Input: part model. Units: mm. Frame: model coordinates. A direction names the side the tool comes from. Round coordinates to 2 decimals unless told otherwise and drop trailing zeros. Write each loop counter-clockwise with the first axis right and the second up, starting at its lowest first coordinate (ties: lowest second). Pieces come first, ordered by that corner, then holes. Notation, with made-up numbers: (0, 6.25) - (47, 6.25) arc R21 cw to (47, 38.25) - close; hole circle Ø11 at (46.5, 14). An arc over 180 degrees is marked (long way). One line per item, written item: value. Start each with the question number.
```python
from build123d import *

# Parameters (mm, degrees)
BOX028_W          = 41.4
BOX028_H          = 10
BOX028_DEPTH      = 11
BOX028_ROLL_ANGLE = 45
BOX037_W          = 0.4
BOX037_H          = 27
BOX037_DEPTH      = 9
BOX036_W          = 0.4
BOX036_H          = 27
BOX036_DEPTH      = 9
BOX035_W          = 0.4
BOX035_H          = 27
BOX035_DEPTH      = 9
BOX034_W          = 0.4
BOX034_H          = 27
BOX034_DEPTH      = 9
BOX038_W          = 0.4
BOX038_H          = 27
BOX038_DEPTH      = 9
BOX033_W          = 36.4
BOX033_H          = 27
BOX033_DEPTH      = 0.4


with BuildPart() as rear_panel_chamfer:
    # Box028 → Box028 (new body)
    with BuildSketch(Plane.XY):
        with Locations((20.7, 5)):
            Rectangle(BOX028_W, BOX028_H)
    extrude(amount=BOX028_DEPTH)


with BuildPart() as rear_panel_chamfer_1:
    # Box028 roll: moved
    add(rear_panel_chamfer.part.rotate(Axis((0, 0, 0), (1, 0, 0)), BOX028_ROLL_ANGLE))


with BuildPart() as rear_panel_chamfer_2:
    # Box028 placement: moved
    add(rear_panel_chamfer_1.part.moved(Location((-21.6, 27, 12.81))))


with BuildPart() as support_y4_for_rear_panel_angled:
    # Box037 → Box037 (new body)
    with BuildSketch(Plane(origin=(-2.2, 0.1, 11.4), x_dir=(1, 0, 0), z_dir=(0, 0, 1))):
        with Locations((0.2, 13.5)):
            Rectangle(BOX037_W, BOX037_H)
    extrude(amount=BOX037_DEPTH)


with BuildPart() as support_y3_for_rear_panel_angled:
    # Box036 → Box036 (new body)
    with BuildSketch(Plane(origin=(4.8, 0.1, 11.4), x_dir=(1, 0, 0), z_dir=(0, 0, 1))):
        with Locations((0.2, 13.5)):
            Rectangle(BOX036_W, BOX036_H)
    extrude(amount=BOX036_DEPTH)


with BuildPart() as support_y2_for_rear_panel_angled:
    # Box035 → Box035 (new body)
    with BuildSketch(Plane(origin=(-8.2, 0.1, 11.4), x_dir=(1, 0, 0), z_dir=(0, 0, 1))):
        with Locations((0.2, 13.5)):
            Rectangle(BOX035_W, BOX035_H)
    extrude(amount=BOX035_DEPTH)


with BuildPart() as support_y1_for_rear_panel_angled:
    # Box034 → Box034 (new body)
    with BuildSketch(Plane(origin=(-14.2, 0.1, 11.4), x_dir=(1, 0, 0), z_dir=(0, 0, 1))):
        with Locations((0.2, 13.5)):
            Rectangle(BOX034_W, BOX034_H)
    extrude(amount=BOX034_DEPTH)


with BuildPart() as support_y5_for_rear_panel_angled:
    # Box038 → Box038 (new body)
    with BuildSketch(Plane(origin=(10.8, 0.1, 11.4), x_dir=(1, 0, 0), z_dir=(0, 0, 1))):
        with Locations((0.2, 13.5)):
            Rectangle(BOX038_W, BOX038_H)
    extrude(amount=BOX038_DEPTH)


with BuildPart() as supports_for_rear_panel_angled_chamfered:
    # Box033 → Box033 (new body)
    with BuildSketch(Plane(origin=(-19, 0.1, 11.4), x_dir=(1, 0, 0), z_dir=(0, 0, 1))):
        with Locations((18.2, 13.5)):
            Rectangle(BOX033_W, BOX033_H)
    extrude(amount=BOX033_DEPTH)

    # Fusion005: union support Y4 for rear panel angled, support Y3 for rear panel angled, support Y2 for rear panel angled, support Y1 for rear panel angled, support Y5 for rear panel angled
    add(support_y4_for_rear_panel_angled.part)
    add(support_y3_for_rear_panel_angled.part)
    add(support_y2_for_rear_panel_angled.part)
    add(support_y1_for_rear_panel_angled.part)
    add(support_y5_for_rear_panel_angled.part)

    # Cut006: cut Rear panel chamfer
    add(rear_panel_chamfer_2.part, mode=Mode.SUBTRACT)


solid = supports_for_rear_panel_angled_chamfered.part
```
Q1. Access query for faces 4 (the flat face through (8, 14, 11.8)), 5 (the flat face through (14, 14, 11.8)), 6 (the flat face through (-0.88, 0.1, 11.55)). Directions: +Z, -Z, +X, -X, +Y, -Y. A direction counts if a zero-diameter tool reaches every point of the face in a straight line with its end or side. Return the directions, or none.
Q2. Pull-direction query (X, two-part tool) for faces 1 (the flat face through (-17, 14, 11.8)), 2 (the flat face through (-11, 14, 11.8)), 3 (the flat face through (11.2, 13, 16)); classes: pulls with the +X half, pulls with the -X half, needs draft (parallel to the pull), parting line crosses it, or undercut.
Q3. Contact query for flat-ended pins moving along their axis: pin 1 Ø4.5 at (y, z) = (13.5, 14.5) entering from +X; pin 2 Ø1.7 at (x, y) = (-10.5, 19.5) entering from +Z; pin 3 Ø5 at (y, z) = (20, 13) entering from -X; pin 4 Ø1.5 at (x, z) = (12, 19) entering from +Y. Output: stop coordinate, or through.
Q4. Cut plane A-A, the plane z = 15.5. Output: boundary loops of the cut face in (x, y), and give its area (3 significant figures).
Q5. Cut plane D-D, the plane y = 17.75. Output: boundary loops of the cut face in (x, z).
Q6. Material intervals for probe 1 along X at (y, z) = (7.5, 15.5); probe 2 along Z at (x, y) = (-6.5, 12.5); probe 3 along Y at (x, z) = (-14, 15), sorted ascending. Write a range as from..to.
Q7. Cut plane B-B, the plane y = 23.25. Output: boundary loops of the cut face in (x, z), and give its area (3 significant figures).
Q8. Cut plane C-C, the plane z = 17.75. Output: boundary loops of the cut face in (x, y), and give its area (3 significant figures).
A:
1. face 4: +Z, +Y, -Y
1. face 5: +Z, +X, +Y, -Y
1. face 6: +Z, -Z, +X, -X, -Y
2. face 1: needs draft
2. face 2: undercut
2. face 3: pulls with the +X half
3. pin 1: stops at x = 11.2
3. pin 2: stops at z = 11.8
3. pin 3: stops at x = -19
3. pin 4: passes through
4. outline: (-14.2, 0.1) - (-13.8, 0.1) - (-13.8, 24.31) - (-14.2, 24.31) - close; (-8.2, 0.1) - (-7.8, 0.1) - (-7.8, 24.31) - (-8.2, 24.31) - close; (-2.2, 0.1) - (-1.8, 0.1) - (-1.8, 24.31) - (-2.2, 24.31) - close; (4.8, 0.1) - (5.2, 0.1) - (5.2, 24.31) - (4.8, 24.31) - close; (10.8, 0.1) - (11.2, 0.1) - (11.2, 24.31) - (10.8, 24.31) - close
4. area: 48.4 mm²
5. outline: (-19, 11.4) - (17.4, 11.4) - (17.4, 11.8) - (11.2, 11.8) - (11.2, 20.4) - (10.8, 20.4) - (10.8, 11.8) - (5.2, 11.8) - (5.2, 20.4) - (4.8, 20.4) - (4.8, 11.8) - (-1.8, 11.8) - (-1.8, 20.4) - (-2.2, 20.4) - (-2.2, 11.8) - (-7.8, 11.8) - (-7.8, 20.4) - (-8.2, 20.4) - (-8.2, 11.8) - (-13.8, 11.8) - (-13.8, 20.4) - (-14.2, 20.4) - (-14.2, 11.8) - (-19, 11.8) - close
6. probe 1: x = -14.2..-13.8, -8.2..-7.8, -2.2..-1.8, 4.8..5.2, 10.8..11.2
6. probe 2: z = 11.4..11.8
6. probe 3: y = 0.1..24.81
7. outline: (-19, 11.4) - (17.4, 11.4) - (17.4, 11.8) - (11.2, 11.8) - (11.2, 16.56) - (10.8, 16.56) - (10.8, 11.8) - (5.2, 11.8) - (5.2, 16.56) - (4.8, 16.56) - (4.8, 11.8) - (-1.8, 11.8) - (-1.8, 16.56) - (-2.2, 16.56) - (-2.2, 11.8) - (-7.8, 11.8) - (-7.8, 16.56) - (-8.2, 16.56) - (-8.2, 11.8) - (-13.8, 11.8) - (-13.8, 16.56) - (-14.2, 16.56) - (-14.2, 11.8) - (-19, 11.8) - close
7. area: 24.1 mm²
8. outline: (-14.2, 0.1) - (-13.8, 0.1) - (-13.8, 22.06) - (-14.2, 22.06) - close; (-8.2, 0.1) - (-7.8, 0.1) - (-7.8, 22.06) - (-8.2, 22.06) - close; (-2.2, 0.1) - (-1.8, 0.1) - (-1.8, 22.06) - (-2.2, 22.06) - close; (4.8, 0.1) - (5.2, 0.1) - (5.2, 22.06) - (4.8, 22.06) - close; (10.8, 0.1) - (11.2, 0.1) - (11.2, 22.06) - (10.8, 22.06) - close
8. area: 43.9 mm²
